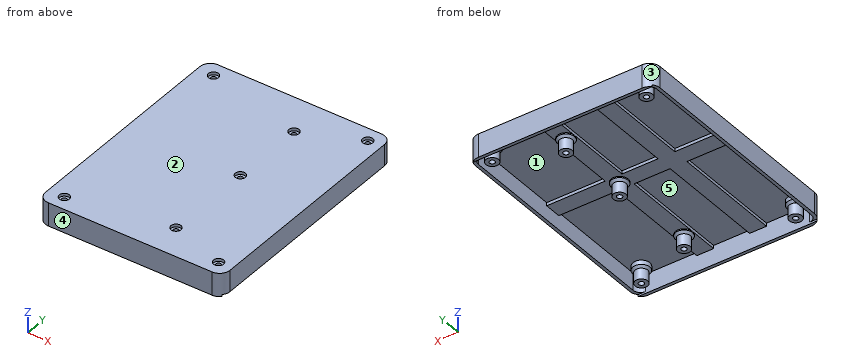
from build123d import *

# Parameters (mm, degrees)
F7_DEPTH        = 8.9
F9_DEPTH        = 0.8
F11_W           = 14.971
F11_H           = 45.903
F11_H_2         = 42.347
F13_DEPTH       = 7.1999999775
F14_DEPTH       = 5.9
F10_R           = 2.6
F16_R           = 3.5
F18_DEPTH       = 4.4
F19_SIZE        = 0.89999
F20_D           = 2.2
F20_CBORE_D     = 4.2
F20_CBORE_DEPTH = 1.2
F21_W           = 84.162
F21_H           = 95.25
F22_DEPTH       = 0.801


# Not quite as in the source:
# - a fillet or chamfer is up to 0.001 mm smaller than in the source, because OpenCascade refuses the exact size


with BuildPart() as f7:
    # F4 (on offset) → F7 (new body, through all)
    with BuildSketch(Plane.XY.offset(1.7)):
        with BuildLine():
            Line((84.612, 3), (84.612, 92.25))
            ThreePointArc((84.612, 92.25), (83.3525591591, 95.2905591591), (80.312, 96.55))
            Line((80.312, 96.55), (12.15, 96.55))
            ThreePointArc((12.15, 96.55), (9.1094408409, 95.2905591591), (7.85, 92.25))
            Line((7.85, 92.25), (7.85, 3))
            ThreePointArc((7.85, 3), (9.1094408409, -0.0405591591), (12.15, -1.3))
            Line((12.15, -1.3), (80.312, -1.3))
            ThreePointArc((80.312, -1.3), (83.3525591591, -0.0405591591), (84.612, 3))
        make_face()
    extrude(amount=F7_DEPTH)

    # F8 (on offset) → F9 (join)
    with BuildSketch(Plane.XY.offset(1.7)):
        with BuildLine():
            Line((84.612, 3), (84.612, 92.25))
            ThreePointArc((84.612, 92.25), (83.3525591591, 95.2905591591), (80.312, 96.55))
            Line((80.312, 96.55), (12.15, 96.55))
            ThreePointArc((12.15, 96.55), (9.1094408409, 95.2905591591), (7.85, 92.25))
            Line((7.85, 92.25), (7.85, 3))
            ThreePointArc((7.85, 3), (9.1094408409, -0.0405591591), (12.15, -1.3))
            Line((12.15, -1.3), (80.312, -1.3))
            ThreePointArc((80.312, -1.3), (83.3525591591, -0.0405591591), (84.612, 3))
        make_face()
        with BuildLine():
            ThreePointArc((80.312, 95.25), (82.4333203436, 94.3713203436), (83.312, 92.25))
            Line((83.312, 92.25), (83.312, 3))
            ThreePointArc((83.312, 3), (82.4333203436, 0.8786796564), (80.312, 0))
            Line((80.312, 0), (12.15, 0))
            ThreePointArc((12.15, 0), (10.0286796564, 0.8786796564), (9.15, 3))
            Line((9.15, 3), (9.15, 92.25))
            ThreePointArc((9.15, 92.25), (10.0286796564, 94.3713203436), (12.15, 95.25))
            Line((12.15, 95.25), (80.312, 95.25))
        make_face(mode=Mode.SUBTRACT)
    extrude(amount=-F9_DEPTH)

    # F11 (on offset) → F13 (cut, through all)
    with BuildSketch(Plane.XY.offset(1.7)):
        with BuildLine():
            Line((58.999, 0), (80.312, 0))
            ThreePointArc((80.312, 0), (82.4333203436, 0.8786796564), (83.312, 3))
            Line((83.312, 3), (83.312, 45.903))
            Line((83.312, 45.903), (58.999, 45.903))
            Line((58.999, 45.903), (58.999, 0))
        make_face()
        with Locations((44.5135, 22.9515)):
            Rectangle(F11_W, F11_H)
        with BuildLine():
            Line((9.15, 45.903), (9.15, 3))
            ThreePointArc((9.15, 3), (10.0286796564, 0.8786796564), (12.15, 0))
            Line((12.15, 0), (30.028, 0))
            Line((30.028, 0), (30.028, 45.903))
            Line((30.028, 45.903), (9.15, 45.903))
        make_face()
        with Locations((44.5135, 74.0765)):
            Rectangle(F11_W, F11_H_2)
        with BuildLine():
            Line((80.312, 95.25), (58.999, 95.25))
            Line((58.999, 95.25), (58.999, 52.903))
            Line((58.999, 52.903), (83.312, 52.903))
            Line((83.312, 52.903), (83.312, 92.25))
            ThreePointArc((83.312, 92.25), (82.4333203436, 94.3713203436), (80.312, 95.25))
        make_face()
        with BuildLine():
            ThreePointArc((12.15, 95.25), (10.0286796564, 94.3713203436), (9.15, 92.25))
            Line((9.15, 92.25), (9.15, 52.903))
            Line((9.15, 52.903), (30.028, 52.903))
            Line((30.028, 52.903), (30.028, 95.25))
            Line((30.028, 95.25), (12.15, 95.25))
        make_face()
    extrude(amount=F13_DEPTH, mode=Mode.SUBTRACT)

    # F8 (on offset) → F14 (cut, through all)
    with BuildSketch(Plane.XY.offset(1.7)):
        with BuildLine():
            Line((83.312, 3), (83.312, 92.25))
            ThreePointArc((83.312, 92.25), (82.4333203436, 94.3713203436), (80.312, 95.25))
            Line((80.312, 95.25), (12.15, 95.25))
            ThreePointArc((12.15, 95.25), (10.0286796564, 94.3713203436), (9.15, 92.25))
            Line((9.15, 92.25), (9.15, 3))
            ThreePointArc((9.15, 3), (10.0286796564, 0.8786796564), (12.15, 0))
            Line((12.15, 0), (80.312, 0))
            ThreePointArc((80.312, 0), (82.4333203436, 0.8786796564), (83.312, 3))
        make_face()
    extrude(amount=F14_DEPTH, mode=Mode.SUBTRACT)

    # F10 (on offset) → F15 (join, up to the next surface of F7)
    with BuildSketch(Plane.XY.offset(1.7)):
        with Locations((78.74, 90.678)):
            Circle(F10_R)
        with Locations((55.499, 80.3793147206)):
            Circle(F10_R)
        with Locations((14.608, 90.678)):
            Circle(F10_R)
        with Locations((55.499, 49.403)):
            Circle(F10_R)
        with Locations((14.608, 4.572)):
            Circle(F10_R)
        with Locations((55.499, 12.2474404052)):
            Circle(F10_R)
        with Locations((78.74, 4.572)):
            Circle(F10_R)
    extrude(until=Until.NEXT)

    # F16 (on offset) → F18 (join, through all)
    with BuildSketch(Plane.XY.offset(10.6)):
        with Locations((78.74, 4.572)):
            Circle(F16_R)
        with Locations((78.74, 90.678)):
            Circle(F16_R)
        with Locations((55.499, 80.3793147206)):
            Circle(F16_R)
        with Locations((55.499, 12.2474404052)):
            Circle(F16_R)
        with Locations((14.608, 90.678)):
            Circle(F16_R)
        with Locations((14.608, 4.572)):
            Circle(F16_R)
        with Locations((55.499, 49.403)):
            Circle(F16_R)
    extrude(amount=-F18_DEPTH)

    # F19 (size 0.9 in the source; OpenCascade refuses exactly that, so slightly less here)
    f19_edges = [f7.edges().sort_by_distance(p)[0] for p in [
        (75.24, 90.678, 6.2),
        (51.999, 80.379315, 6.2),
        (11.108, 90.678, 6.2),
        (51.999, 49.403, 6.2),
        (51.999, 12.24744, 6.2),
        (75.24, 4.572, 6.2),
        (11.108, 4.572, 6.2),
    ]]
    chamfer(f19_edges, length=F19_SIZE)

    # F20 (through all)
    with Locations(Plane.XY.offset(10.6)):
        with Locations((78.74, 90.678), (55.499, 80.3793147206), (55.499, 49.403), (14.608, 90.678), (55.499, 12.2474404052), (78.74, 4.572), (14.608, 4.572)):
            CounterBoreHole(F20_D / 2, F20_CBORE_D / 2, F20_CBORE_DEPTH)

    # F21 (on offset) → F22 (cut, through all)
    with BuildSketch(Plane.XY.offset(1.7)):
        with Locations((46.231, 47.625)):
            Rectangle(F21_W, F21_H)
    extrude(amount=-F22_DEPTH, mode=Mode.SUBTRACT)


solid = f7.part
Could you check a few things on this model? Use its own coordinates, in mm. Face numbers are marked on the shaded views. A direction names the side the tool comes from. Give positions to 0.01 mm unless a question says otherwise; leave off trailing zeros. Loops run counter-clockwise (first coordinate to the right, second up) from the corner with the lowest first, then second, coordinate; pieces in that order, holes last. Notation, with made-up numbers: (42.5, 78) -> (71.5, 78) arc R34 ccw to (71.5, 112) -> close; hole circle Ø10 at (33, 45). An arc over 180 degrees is marked (long way). Answer as CSV lines item,"result". Start each with the question number.
(1) I need wall thicknesses on probe 1 along Y at (x, z) = (73, 8.25); probe 2 along X at (y, z) = (26, 4); probe 3 along Y at (x, z) = (21.5, 2.5). Which ranges of each line are inside material? Lowest first, please.
(2) If we section it at C-C on x = 66: Write out the boundary of the cut face in (y, z), then the cut area to 3 significant figures.
(3) If we section it at A-A on y = 22: Write out the boundary of the cut face in (x, z).
(4) Which directions (+Z, -Z, +X, -X, +Y, -Y) give clear straight access to the entire face, cutting with the end or side of a thin tool? Please do the marked faces 1 and 2.
(5) I'm going to push flat-ended pins straight in: pin 1 Ø2.5 at (x, y) = (14.608, 90.678) entering from -Z; pin 2 Ø12 at (x, y) = (62.5, 42) entering from -Z; pin 3 Ø6.5 at (x, y) = (23.5, 21) entering from -Z; pin 4 Ø3.5 at (x, y) = (15, 91) entering from +Z. Where does each tip first touch, or does it pass through?
(6) If we section it at B-B on z = 5: Count the separate pieces of the cut face and the enclosed holes in it, then the cut area to 3 significant figures.
(7) We'd pull the mould along Y, two halves only. Please class the marked faces 3, 4 and 5: released by +Y, released by -Y, zero draft, split by the parting line, or undercut.
Computed:
1,probe 1,"y = -1.3 to 0, 45.9 to 52.9, 95.25 to 96.55"
1,probe 2,"x = 7.85 to 9.15, 83.31 to 84.61"
1,probe 3,"y = -1.3 to 0, 95.25 to 96.55"
2,outline,"(-1.3, 0.9) -> (0, 0.9) -> (0, 8.9) -> (45.9, 8.9) -> (45.9, 7.6) -> (52.9, 7.6) -> (52.9, 8.9) -> (95.25, 8.9) -> (95.25, 0.9) -> (96.55, 0.9) -> (96.55, 10.6) -> (-1.3, 10.6) -> close"
2,area,"196 mm2"
3,outline,"(7.85, 1.7) -> (9.15, 1.7) -> (9.15, 8.9) -> (30.03, 8.9) -> (30.03, 7.6) -> (37.03, 7.6) -> (37.03, 8.9) -> (52, 8.9) -> (52, 7.6) -> (59, 7.6) -> (59, 8.9) -> (83.31, 8.9) -> (83.31, 1.7) -> (84.61, 1.7) -> (84.61, 10.6) -> (7.85, 10.6) -> close"
4,face 1,"-Z"
4,face 2,"+Z, +X, -X, +Y, -Y"
5,pin 1,"stops at z = 1.7"
5,pin 2,"stops at z = 7.6"
5,pin 3,"stops at z = 8.9"
5,pin 4,"stops at z = 10.6"
6,separate pieces,"8"
6,enclosed holes,"8"
6,area,"561 mm2"
7,face 3,"released by +Y"
7,face 4,"released by -Y"
7,face 5,"undercut"
